```python
from build123d import *

# Parameters (mm, degrees)
SKETCH2_R          = 7.5
CUT_EXTRUDE1_DEPTH = 27.038433133
SKETCH3_R          = 2
CUT_EXTRUDE2_DEPTH = 27


with BuildPart() as part:
    # Sketch1 → Revolve1 (revolve)
    with BuildSketch(Plane(origin=(0, 0, 0), x_dir=(1, 0, 0), z_dir=(0, 1, 0)), mode=Mode.PRIVATE) as revolve1_sk:
        Polygon((0, 0), (17, 0), (17, 1), (16, 1), (16, 9), (17, 9), (17, 10), (0, 10), align=None)
    revolve(revolve1_sk.sketch.rotate(Axis((0, 0, -10), (0, 0, 1)), 180), axis=Axis((0, 0, -10), (0, 0, 1)))

    # Sketch2 → Cut-Extrude1 (cut, through all)
    with BuildSketch(Plane(origin=(0, 0, -10), x_dir=(-1, 0, 0), z_dir=(0, 0, -1))):
        Circle(SKETCH2_R)
    extrude(amount=-CUT_EXTRUDE1_DEPTH, mode=Mode.SUBTRACT)

    # Sketch3 → Cut-Extrude2 (cut)
    with BuildSketch(Plane(origin=(0, 0, 0), x_dir=(1, 0, 0), z_dir=(0, 1, 0))):
        with Locations(Location((0, 5, 0), (0, 0, 270))):
            Circle(SKETCH3_R)
    extrude(amount=-CUT_EXTRUDE2_DEPTH, mode=Mode.SUBTRACT)


solid = part.part
```
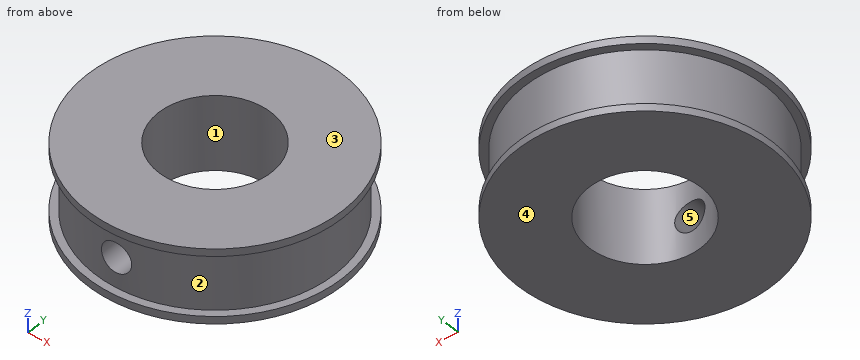
Verification items for the finished model (mm, model axes). Face numbers are marked on the shaded views. A direction names the side the tool comes from. Give positions to 0.01 mm unless a question says otherwise; leave off trailing zeros. Order: outer loops, then holes, each group sorted by start corner. A loop starts at its lowest first (then second) coordinate and runs counter-clockwise, first axis right, second up. Notation, with made-up numbers: M 15,-21 L 41,-21 A14 ccw 41,-5 Z; hole C -35.75,19.25 d8. An arc over 180 degrees is marked long. Return JSON: item names as keys, results as strings. Group by question number.
1) Go/stop test with flat-tipped pins: pin 1 Ø5 at (x, z) = (-0.5, -5.5) entering from -Y; pin 2 Ø6 at (x, z) = (-6.5, -7) entering from -Y; pin 3 Ø1 at (y, z) = (-5.5, -7) entering from +X. Record where each tip stops, or that it passes through.
2) Section check A-A on x = 0. Record the cut outline in (y, z).
3) Section check D-D on x = -9. Record the cut outline in (y, z), and give its area (3 significant figures).
4) Section check C-C on z = -2.5. Record the cut outline in (x, y).
5) Mould release check, pull along Y, two halves, no side actions. Record for the marked faces 1, 2 and 3: pulls with the +Y half, pulls with the -Y half, needs draft (parallel to the pull), parting line crosses it, or undercut.
6) Section check B-B on y = 0. Record the cut outline in (x, z), and give its area (3 significant figures).
7) Access from +Z, -Z, +X, -X, +Y, -Y to the whole of each face (thin tool, end or side, straight path). Record for the marked faces 4 and 5.
8) Scan lines: line 1 (Z direction, x = 0, y = -11); line 2 (Y direction, x = 0, z = -2.5); line 3 (Y direction, x = 0, z = -3.75). Record each from-to range of solid material in increasing order.
Answer block:
{
 "1": {"pin 1": "stops at y = -16", "pin 2": "stops at y = -16.46", "pin 3": "stops at x = 15.2"},
 "2": {"outline": "M -17,-10 L -7.5,-10 L -7.5,-7 L -16,-7 L -16,-9 L -17,-9 Z; M -17,-1 L -16,-1 L -16,-3 L -7.5,-3 L -7.5,0 L -17,0 Z; M 7.5,-10 L 17,-10 L 17,-9 L 16,-9 L 16,-1 L 17,-1 L 17,0 L 7.5,0 Z"},
 "3": {"outline": "M -14.42,-10 L 14.42,-10 L 14.42,-9 L 13.23,-9 L 13.23,-1 L 14.42,-1 L 14.42,0 L -14.42,0 L -14.42,-1 L -13.23,-1 L -13.23,-9 L -14.42,-9 Z", "area": "269 mm^2"},
 "4": {"outline": "C 0,0 d32; hole C 0,0 d15"},
 "5": {"face 1": "undercut", "face 2": "parting line crosses it", "face 3": "needs draft"},
 "6": {"outline": "M -17,-10 L -7.5,-10 L -7.5,0 L -17,0 L -17,-1 L -16,-1 L -16,-9 L -17,-9 Z; M 7.5,-10 L 17,-10 L 17,-9 L 16,-9 L 16,-1 L 17,-1 L 17,0 L 7.5,0 Z", "area": "174 mm^2"},
 "7": {"face 4": "-Z, +X, -X, +Y, -Y", "face 5": "-Y"},
 "8": {"line 1": "z = -10 to -7, -3 to 0", "line 2": "y = -16 to -7.5, 7.5 to 16", "line 3": "y = 7.5 to 16"}
}
